```python
from build123d import *

# Parameters (mm, degrees)
BOSS_EXTRUDE1_DEPTH    = 50
SKETCH2_R              = 5.5
SKETCH2_R_2            = 1.5
CUT_EXTRUDE1_DEPTH     = 50
SKETCH3_R              = 2.5
CUT_EXTRUDE3_DEPTH     = 10
CONVERT_SOLID1_DEPTH   = 50
CONVERT_SOLID1_2_DEPTH = 50
FILLET1_R              = 4


# Read off the part's stored shape, not the designer's step: Convert-Solid1
with BuildPart() as part:
    # Sketch1 → Boss-Extrude1 (new body)
    with BuildSketch(Plane(origin=(0, 0, 0), x_dir=(0, 0, -1), z_dir=(1, 0, 0))):
        Polygon((0, 0), (0, -60), (-21, -60), (-21, -30), (-17, -30), (-17, -56), (-4, -56), (-4, 0), align=None)
    extrude(amount=BOSS_EXTRUDE1_DEPTH)

    # Sketch2 → Cut-Extrude1 (cut)
    with BuildSketch(Plane.XY.offset(4)):
        with Locations((25, -15)):
            Circle(SKETCH2_R)
        with Locations((25, -6)):
            Circle(SKETCH2_R_2)
        with Locations((16, -15)):
            Circle(SKETCH2_R_2)
        with Locations((25, -24)):
            Circle(SKETCH2_R_2)
        with Locations((34, -15)):
            Circle(SKETCH2_R_2)
    extrude(amount=-CUT_EXTRUDE1_DEPTH, mode=Mode.SUBTRACT)

    # Sketch3 → Cut-Extrude3 (cut)
    with BuildSketch(Plane.XY.offset(21)):
        with Locations((12.5, -45)):
            Circle(SKETCH3_R)
        with Locations((37.5, -45)):
            Circle(SKETCH3_R)
    extrude(amount=-CUT_EXTRUDE3_DEPTH, mode=Mode.SUBTRACT)

    # Convert-Solid1 outline → Convert-Solid1 (cut)
    with BuildSketch(Plane.YZ):
        with BuildLine():
            Line((-60, 21), (-60, 13))
            ThreePointArc((-60, 13), (-57.656854249, 18.656854249), (-52, 21))
            Line((-52, 21), (-60, 21))
        make_face()
        with BuildLine():
            ThreePointArc((-52, 0), (-57.656854249, 2.343145751), (-60, 8))
            Line((-60, 8), (-60, 0))
            Line((-60, 0), (-52, 0))
        make_face()
    extrude(amount=CONVERT_SOLID1_DEPTH, mode=Mode.SUBTRACT)

    # Convert-Solid1 2 outline → Convert-Solid1 2 (add)
    with BuildSketch(Plane.YZ):
        with BuildLine():
            ThreePointArc((-52, 4), (-54.828427125, 5.171572875), (-56, 8))
            Line((-56, 8), (-56, 4))
            Line((-56, 4), (-52, 4))
        make_face()
        with BuildLine():
            Line((-56, 17), (-56, 13))
            ThreePointArc((-56, 13), (-54.828427125, 15.828427125), (-52, 17))
            Line((-52, 17), (-56, 17))
        make_face()
    extrude(amount=CONVERT_SOLID1_2_DEPTH)

    # Fillet1
    fillet1_edges = [part.edges().sort_by_distance(p)[0] for p in [
        (50, -30, 19),
        (0, -30, 19),
        (0, 0, 2),
        (50, 0, 2),
    ]]
    fillet(fillet1_edges, radius=FILLET1_R)


solid = part.part
```
Can you work these out from the model? Positions are in its coordinate system, mm. A direction names the side the tool comes from. Round coordinates to 2 decimals unless told otherwise and drop trailing zeros. Loops run counter-clockwise (first coordinate to the right, second up) from the corner with the lowest first, then second, coordinate; pieces in that order, holes last. Notation, with made-up numbers: M 38,3 L 94,3 A27 cw 94,29 Z; hole C 86.5,40 d7. An arc over 180 degrees is marked long. Write item = value, one per line. Start each with the question number.
(1) Suppose I cut it at D-D on x = 5. Write out the boundary of the cut face in (y, z).
(2) If we mould it in two halves opening along Y, with no side actions, what happens to faces 4 (the face through (25, -26, 0)), 5 (the face through (25, -56, 11)), 6 (the face through (23.89, -22.99, 2.03)), 7 (the face through (11.96, -47.44, 19.03))? For each: released by +Y, released by -Y, zero draft, split by the parting line, or undercut.
(3) I need wall thicknesses on line 1 along Z through (x, y) = (48.5, -42.5); line 2 along Y through (x, z) = (25, 1.7); line 3 along Y through (x, z) = (25, 2.3). Which ranges of each line are inside material? Lowest first, please.
(4) Suppose I cut it at C-C on y = -45. Write out the boundary of the cut face in (x, z), plus the area to 3 significant figures.
(5) I'm going to push flat-ended pins straight in: P1, Ø9, axis at x = 25, y = -15, coming from the +Z side; P2, Ø3.5, axis at x = 16, y = -15, coming from the +Z side; P3, Ø4.5, axis at x = 20.5, z = 20, coming from the +Y side; P4, Ø4, axis at x = 29, z = 11, coming from the +Y side. Where does each tip first touch, or does it pass through?
(6) Which directions (+Z, -Z, +X, -X, +Y, -Y) give clear straight access to the entire face, cutting with the end or side of a thin tool? Please do faces 1 (the face through (24.65, -54.859, 15.797)), 2 (the face through (1.141, -31.203, 18.972)), 3 (the face through (25, -30, 19)).
(7) Suppose I cut it at A-A on y = -35. Write out the boundary of the cut face in (x, z), plus the area to 3 significant figures.
(8) Suppose I cut it at B-B on x = 12.5. Write out the boundary of the cut face in (y, z).
Answer block:
q1.outline = M -60,8 A8 ccw -52,0 L 0,0 L 0,4 L -52,4 A4 cw -56,8 L -56,13 A4 cw -52,17 L -30,17 L -30,21 L -52,21 A8 ccw -60,13 Z
q2.face_4 = zero draft
q2.face_5 = released by +Y
q2.face_6 = undercut
q2.face_7 = undercut
q3.line_1 = 0 to 4, 17 to 21
q3.line_2 = -56.93 to -25.5, -22.5 to -20.5, -9.5 to -7.5, -4.5 to 0
q3.line_3 = -57.61 to -25.5, -22.5 to -20.5, -9.5 to -7.5, -4.5 to 0
q4.outline = M 0,0 L 50,0 L 50,4 L 0,4 Z; M 0,17 L 10,17 L 10,21 L 0,21 Z; M 15,17 L 35,17 L 35,21 L 15,21 Z; M 40,17 L 50,17 L 50,21 L 40,21 Z
q4.area = 360 mm²
q5.P1 = through
q5.P2 = 4
q5.P3 = -30
q5.P4 = -56
q6.face_1 = +X, -X, +Y
q6.face_2 = +Z, -X, +Y
q6.face_3 = +Z, +X, -X, +Y
q7.outline = M 0,0 L 50,0 L 50,4 L 0,4 Z; M 0,17 L 50,17 L 50,21 L 0,21 Z
q7.area = 400 mm²
q8.outline = M -60,8 A8 ccw -52,0 L 0,0 L 0,4 L -52,4 A4 cw -56,8 L -56,13 A4 cw -52,17 L -47.5,17 L -47.5,21 L -52,21 A8 ccw -60,13 Z; M -42.5,17 L -30,17 L -30,21 L -42.5,21 Z
